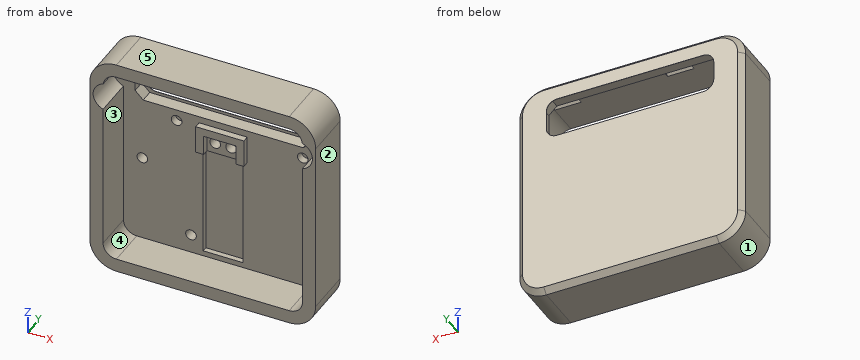
from build123d import *

# Parameters (mm, degrees)
SKETCH1_W           = 85
SKETCH1_H           = 85
BOSS_EXTRUDE1_DEPTH = 20
FILLET1_R           = 10
CHAMFER1_SIZE       = 2
SHELL2_T            = -5
CUT_EXTRUDE1_DEPTH  = 64.344297297
SKETCH3_W           = 15
SKETCH3_H           = 41.8
CUT_EXTRUDE2_DEPTH  = 2
SKETCH3_4_R         = 2
CUT_EXTRUDE3_DEPTH  = 4
BOSS_EXTRUDE2_DEPTH = 0.1
CUT_EXTRUDE9_START  = -15
CUT_EXTRUDE9_DEPTH  = 15
SKETCH17_W          = 10
SKETCH17_H          = 1
CUT_EXTRUDE10_DEPTH = 2
CHAMFER4_SIZE       = 2
SKETCH18_R          = 2
CUT_EXTRUDE11_DEPTH = 3
SKETCH19_W          = 12.1
SKETCH19_H          = 3
BOSS_EXTRUDE8_DEPTH = 2.5
SKETCH20_R          = 2
CUT_EXTRUDE12_DEPTH = 4


with BuildPart() as part:
    # Sketch1 → Boss-Extrude1 (new body)
    with BuildSketch(Plane(origin=(0, 0, 0), x_dir=(1, 0, 0), z_dir=(0, 1, 0))):
        Rectangle(SKETCH1_W, SKETCH1_H)
    extrude(amount=BOSS_EXTRUDE1_DEPTH)

    # Fillet1
    fillet1_edges = [part.edges().sort_by_distance(p)[0] for p in [
        (42.5, 10, 42.5),
        (-42.5, 10, 42.5),
        (-42.5, 10, -42.5),
        (42.5, 10, -42.5),
    ]]
    fillet(fillet1_edges, radius=FILLET1_R)

    # Chamfer1
    chamfer1_edges = [part.edges().sort_by_distance(p)[0] for p in [
        (-42.5, 20, 0),
        (0, 20, -42.5),
        (42.5, 20, 0),
        (0, 20, 42.5),
        (-39.571067812, 20, 39.571067812),
        (39.571067812, 20, 39.571067812),
        (39.571067812, 20, -39.571067812),
        (-39.571067812, 20, -39.571067812),
    ]]
    chamfer(chamfer1_edges, length=CHAMFER1_SIZE)

    # Shell2
    shell2_openings = [part.faces().sort_by_distance(p)[0] for p in [
        (0, 0, 0),
    ]]
    offset(amount=SHELL2_T, openings=shell2_openings, kind=Kind.INTERSECTION)

    # Sketch2 → Cut-Extrude1 (cut, through all)
    with BuildSketch(Plane(origin=(0, 20, 0), x_dir=(1, 0, 0), z_dir=(0, 1, 0))):
        Polygon((-30.1, -36.5), (30.1, -36.5), (33.1, -33.5), (33.1, -22.3), (30.1, -19.3), (-30.1, -19.3), (-33.1, -22.3), (-33.1, -33.5), align=None)
    extrude(amount=-CUT_EXTRUDE1_DEPTH, mode=Mode.SUBTRACT)

    # Sketch3 → Cut-Extrude2 (cut)
    with BuildSketch(Plane.XZ.offset(-15)):
        with Locations((0, -14.6)):
            Rectangle(SKETCH3_W, SKETCH3_H)
    extrude(amount=-CUT_EXTRUDE2_DEPTH, mode=Mode.SUBTRACT)

    # Sketch3<4> → Cut-Extrude3 (cut)
    with BuildSketch(Plane.XZ.offset(-15)):
        with Locations(Location((-3, 10.3, 0), (0, 0, 270))):
            Circle(SKETCH3_4_R)
        with Locations(Location((3, 10.3, 0), (0, 0, 270))):
            Circle(SKETCH3_4_R)
    extrude(amount=-CUT_EXTRUDE3_DEPTH, mode=Mode.SUBTRACT)

    # Sketch4 → Boss-Extrude2 (add)
    with BuildSketch(Plane(origin=(0, 20, 0), x_dir=(1, 0, 0), z_dir=(0, 1, 0))):
        Polygon((-33.1, -33.5), (-33.1, -22.3), (-30.1, -19.3), (30.1, -19.3), (33.1, -22.3), (33.1, -33.5), (30.1, -36.5), (-30.1, -36.5), align=None)
        with BuildLine():
            Line((-31.5, -31.4), (-31.5, -24.4))
            ThreePointArc((-31.5, -24.4), (-30.328427125, -21.571572875), (-27.5, -20.4))
            Line((-27.5, -20.4), (27.5, -20.4))
            ThreePointArc((27.5, -20.4), (30.328427125, -21.571572875), (31.5, -24.4))
            Line((31.5, -24.4), (31.5, -31.4))
            ThreePointArc((31.5, -31.4), (30.328427125, -34.228427125), (27.5, -35.4))
            Line((27.5, -35.4), (-27.5, -35.4))
            ThreePointArc((-27.5, -35.4), (-30.328427125, -34.228427125), (-31.5, -31.4))
        make_face(mode=Mode.SUBTRACT)
    extrude(amount=-BOSS_EXTRUDE2_DEPTH)

    # Sketch5 → Cut-Extrude9 (cut)
    with BuildSketch(Plane.XZ.offset(CUT_EXTRUDE9_START)):
        with BuildLine():
            ThreePointArc((-37.460499109, 33.127254805), (-41.249960643, 27.920806881), (-37.5, 22.685836596))
            Line((-37.5, 22.685836596), (-37.5, 32.5))
            ThreePointArc((-37.5, 32.5), (-37.490115006, 32.814248672), (-37.460499109, 33.127254805))
        make_face()
        with BuildLine():
            Line((37.5, 32.5), (37.5, 22.685836596))
            ThreePointArc((37.5, 22.685836596), (41.249960643, 27.920806881), (37.460499109, 33.127254805))
            ThreePointArc((37.460499109, 33.127254805), (37.490115006, 32.814248672), (37.5, 32.5))
        make_face()
    extrude(amount=CUT_EXTRUDE9_DEPTH, mode=Mode.SUBTRACT)

    # Sketch17 → Cut-Extrude10 (cut)
    with BuildSketch(Plane(origin=(0, 0, 37.5), x_dir=(-1, 0, 0), z_dir=(0, 0, -1))):
        with Locations((-27.460499109, 14.5)):
            Rectangle(SKETCH17_W, SKETCH17_H)
        with Locations((15, 14.5)):
            Rectangle(SKETCH17_W, SKETCH17_H)
    extrude(amount=-CUT_EXTRUDE10_DEPTH, mode=Mode.SUBTRACT)

    # Chamfer4
    chamfer4_edges = [part.edges().sort_by_distance(p)[0] for p in [
        (27.460499109, 14, 37.5),
        (-15, 14, 37.5),
    ]]
    chamfer(chamfer4_edges, length=CHAMFER4_SIZE - 0.0001)  # a hair under: the kernel refuses the full size

    # Sketch18 → Cut-Extrude11 (cut)
    with BuildSketch(Plane.XZ.offset(-15)):
        with Locations(Location((-17.5, 15, 0), (0, 0, 270))):
            Circle(SKETCH18_R)
        with Locations(Location((29.960499109, 15, 0), (0, 0, 270))):
            Circle(SKETCH18_R)
    extrude(amount=-CUT_EXTRUDE11_DEPTH, mode=Mode.SUBTRACT)

    # Sketch19 → Boss-Extrude8 (add)
    with BuildSketch(Plane.XZ.offset(-15)):
        with Locations((0, 15.3)):
            Rectangle(SKETCH19_W, SKETCH19_H)
        Polygon((-6.05, 6.3), (-6.05, 13.8), (-6.05, 16.8), (-9.05, 16.8), (-9.05, 6.3), align=None)
        Polygon((6.05, 16.8), (6.05, 13.8), (6.05, 6.3), (9.05, 6.3), (9.05, 16.8), align=None)
    extrude(amount=BOSS_EXTRUDE8_DEPTH)

    # Sketch20 → Cut-Extrude12 (cut)
    with BuildSketch(Plane.XZ.offset(-15)):
        with Locations(Location((-30.4, -4.6, 0), (0, 0, 270))):
            Circle(SKETCH20_R)
        with Locations(Location((-12.1, -30.4, 0), (0, 0, 270))):
            Circle(SKETCH20_R)
    extrude(amount=-CUT_EXTRUDE12_DEPTH, mode=Mode.SUBTRACT)


solid = part.part
Design review of the part built by this model. Coordinates are the model's own, in mm. Face numbers are marked on the shaded views. A direction names the side the tool comes from. Round coordinates to 2 decimals unless told otherwise and drop trailing zeros. Write each loop counter-clockwise with the first axis right and the second up, starting at its lowest first coordinate (ties: lowest second). Pieces come first, ordered by that corner, then holes. Notation, with made-up numbers: (66, 54.5) -> (125, 54.5) arc R32 cw to (125, 88.5) -> close; hole circle Ø6 at (42.25, 73). An arc over 180 degrees is marked (long way). One line per question, with ' | ' between items.
(1) Draft analysis for pull direction Z (two halves, no side actions). For the marked faces 1, 2 and 3, state which applies: released by +Z, released by -Z, zero draft, split by the parting line, or undercut.
Result sheet:
face 1: released by -Z | face 2: zero draft | face 3: undercut
(2) Wall thickness on line 1 (X direction, y = 16.45, z = 10.3); line 2 (X direction, y = 16.75, z = 15); line 3 (X direction, y = 8.75, z = 16.5): over which ranges is each line inside the solid? List them lowest first. Write a range as [from, to].
Result sheet:
line 1: [-42.5, -5], [-1, 1], [5, 42.5] | line 2: [-42.5, -19.5], [-15.5, 27.96], [31.96, 42.5] | line 3: [-42.5, -37.5], [37.5, 42.5]
(3) Take a section at C-C, the plane y = 8. State the section outline as (x, z) points, and give its area (3 significant figures).
Result sheet:
outline: (-42.5, -32.5) arc R10 ccw to (-32.5, -42.5) -> (32.5, -42.5) arc R10 ccw to (42.5, -32.5) -> (42.5, 32.5) arc R10 ccw to (32.5, 42.5) -> (-32.5, 42.5) arc R10 ccw to (-42.5, 32.5) -> close; hole (-37.5, -32.5) arc R5 ccw to (-32.5, -37.5) -> (32.5, -37.5) arc R5 ccw to (37.5, -32.5) -> (37.5, 22.69) arc R5.5 ccw to (37.46, 33.13) arc R5 ccw to (32.5, 37.5) -> (-32.5, 37.5) arc R5 ccw to (-37.46, 33.13) arc R5.5 ccw to (-37.5, 22.69) -> close | area: 1,480 mm2
(4) Machinability: for the marked faces 4 and 5, which of the approach directions +Z, -Z, +X, -X, +Y, -Y give a long, thin tool a straight path to every point of the face, cutting with its end or side? Answer none if there is none.
Result sheet:
face 4: -Y | face 5: +Z, +X, -X, +Y, -Y
(5) Take a section at B-B, the plane z = 15. State the section outline as (x, y) points.
Result sheet:
outline: (-42.5, 0) -> (-37.5, 0) -> (-37.5, 15) -> (-19.5, 15) -> (-19.5, 18) -> (-15.5, 18) -> (-15.5, 15) -> (-9.05, 15) -> (-9.05, 12.5) -> (9.05, 12.5) -> (9.05, 15) -> (27.96, 15) -> (27.96, 18) -> (31.96, 18) -> (31.96, 15) -> (37.5, 15) -> (37.5, 0) -> (42.5, 0) -> (42.5, 18) -> (40.5, 20) -> (-40.5, 20) -> (-42.5, 18) -> close
(6) Insertion check: P1, Ø3, axis at x = 3, z = 10.3, coming from the -Y side; P2, Ø10, axis at x = 9, z = -23.5, coming from the -Y side; P3, Ø1, axis at y = 13.5, z = 38, coming from the +X side. Each pin has a flat end and moves straight along its axis. Give the tip position at first contact, or say it passes through.
Result sheet:
P1: y = 19 | P2: y = 15 | P3: x = 41.16
